Check sheet for the drawn part. Datum: minimum x, y, z corner. Units: mm. Coordinates: 2 decimals unless noted, no trailing zeros. Write each loop counter-clockwise with the first axis right and the second up, starting at its lowest first coordinate (ties: lowest second). Pieces come first, ordered by that corner, then holes. Notation, with made-up numbers: (64.5, 54.25) -> (100.5, 54.25) arc R28 ccw to (100.5, 93.25) -> close; hole circle Ø2 at (-1.5, 51.25). An arc over 180 degrees is marked (long way). Answer in a Markdown table with one row per item. Add a question column.
1. Cross-section at D-D on x = 53. Record the cut outline in (y, z), and give its area (3 significant figures).
2. Depth check by flat-ended pin: P1, Ø0.9, axis at x = 8.5, z = 1.5, coming from the -Y side; P2, Ø1.5, axis at x = 53.5, z = 1, coming from the +Y side; P3, Ø1.5, axis at x = 2, z = 1.5, coming from the +Y side. Enter the tip coordinate at first touch or a pass-through.
3. Cross-section at A-A on y = 55. Record the cut outline in (x, z).
4. Cross-section at C-C on x = 18. Record the cut outline in (y, z).
5. Cross-section at B-B on z = 1.8. Record the cut outline in (x, y).
6. Scan lines: L1, parallel to X at y = 75, z = 1.9; L2, parallel to Y at x = 48.5, z = 0.3; L3, parallel to Y at x = 15, z = 0.9. Record each from-to range of solid material in increasing order. Write a range as from..to.
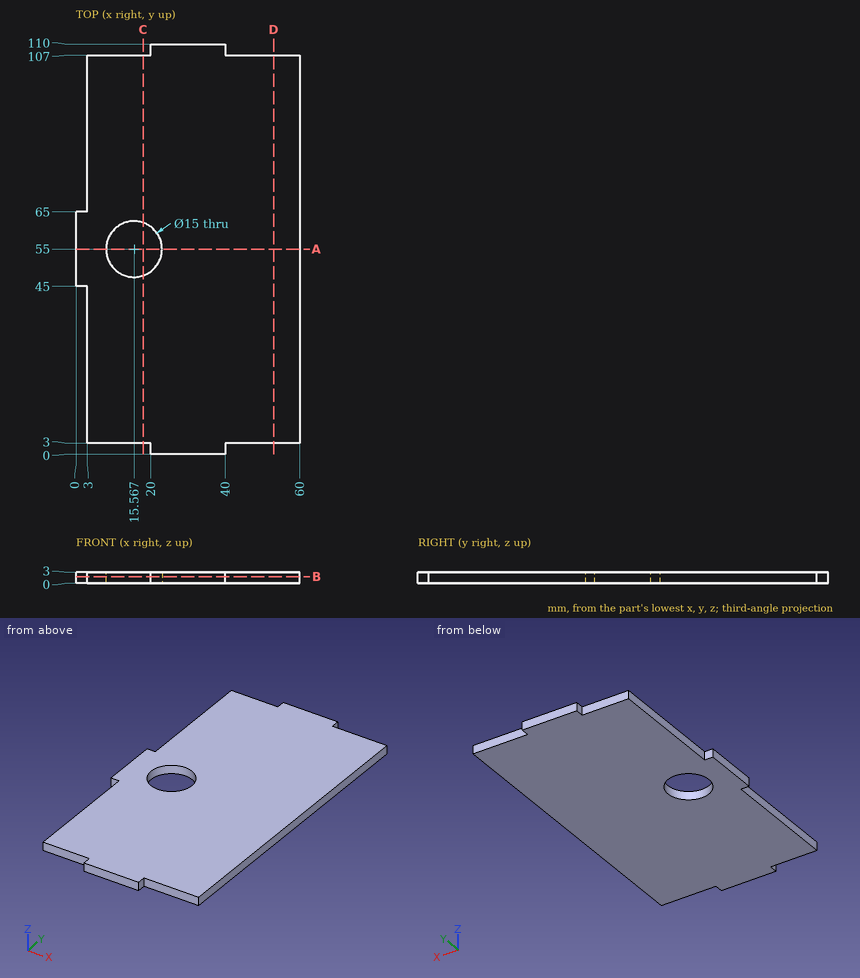
Results found:
| question | item | result |
|---|---|---|
| 1 | outline | (3, 0) -> (107, 0) -> (107, 3) -> (3, 3) -> close |
| 1 | area | 312 mm^2 |
| 2 | P1 | stops at y = 3 |
| 2 | P2 | stops at y = 107 |
| 2 | P3 | stops at y = 65 |
| 3 | outline | (0, 0) -> (8.07, 0) -> (8.07, 3) -> (0, 3) -> close; (23.07, 0) -> (60, 0) -> (60, 3) -> (23.07, 3) -> close |
| 4 | outline | (3, 0) -> (47.91, 0) -> (47.91, 3) -> (3, 3) -> close; (62.09, 0) -> (107, 0) -> (107, 3) -> (62.09, 3) -> close |
| 5 | outline | (0, 45) -> (3, 45) -> (3, 3) -> (20, 3) -> (20, 0) -> (40, 0) -> (40, 3) -> (60, 3) -> (60, 107) -> (40, 107) -> (40, 110) -> (20, 110) -> (20, 107) -> (3, 107) -> (3, 65) -> (0, 65) -> close; hole circle Ø15 at (15.57, 55) |
| 6 | L1 | x = 3..60 |
| 6 | L2 | y = 3..107 |
| 6 | L3 | y = 3..47.52, 62.48..107 |
